from build123d import *

# Parameters (mm, degrees)
F0_R     = 3
F1_DEPTH = 1.5
F2_R     = 7.655
F2_W     = 13
F2_H     = 3
F3_DEPTH = 56.3
F4_R     = 2.93
F5_DEPTH = 26.25
F7_DEPTH = 18
F8_R     = 3
F9_DEPTH = 9.156


with BuildPart() as f1:
    # F0 (on Top) → F1 (new body, symmetric)
    with BuildSketch(Plane.XY):
        with BuildLine():
            Line((-2.85, -6.5), (9.35, -6.5))
            Line((9.35, -6.5), (9.35, 6.5))
            Line((9.35, 6.5), (-2.85, 6.5))
            ThreePointArc((-2.85, 6.5), (-9.35, 0), (-2.85, -6.5))
        make_face()
        with Locations((-2.85, 0)):
            Circle(F0_R, mode=Mode.SUBTRACT)
    extrude(amount=F1_DEPTH, both=True)

    # F2 (on face) → F3 (join)
    with BuildSketch(Plane.YZ.offset(9.35)):
        Circle(F2_R)
        Rectangle(F2_W, F2_H, mode=Mode.SUBTRACT)
        Rectangle(F2_W, F2_H)
    extrude(amount=F3_DEPTH)

    # F4 (on face) → F5 (join)
    with BuildSketch(Plane.YZ.offset(65.65)):
        Circle(F4_R)
    extrude(amount=F5_DEPTH)

    # F6 (on face) → F7 (join)
    with BuildSketch(Plane.YZ.offset(91.9)):
        with BuildLine():
            Line((2.516923, -1.5), (6.44, -1.5))
            Line((6.44, -1.5), (6.44, 1.5))
            Line((6.44, 1.5), (2.516923, 1.5))
            ThreePointArc((2.516923, 1.5), (2.824844, 0.777919), (2.93, 0))
            ThreePointArc((2.93, 0), (2.824844, -0.777919), (2.516923, -1.5))
        make_face()
        with BuildLine():
            Line((-2.516923, -1.5), (2.516923, -1.5))
            ThreePointArc((2.516923, -1.5), (2.824844, -0.777919), (2.93, 0))
            ThreePointArc((2.93, 0), (2.824844, 0.777919), (2.516923, 1.5))
            Line((2.516923, 1.5), (-2.516923, 1.5))
            ThreePointArc((-2.516923, 1.5), (-2.93, 0), (-2.516923, -1.5))
        make_face()
        with BuildLine():
            Line((-6.44, -1.5), (-2.516923, -1.5))
            ThreePointArc((-2.516923, -1.5), (-2.93, 0), (-2.516923, 1.5))
            Line((-2.516923, 1.5), (-6.44, 1.5))
            Line((-6.44, 1.5), (-6.44, -1.5))
        make_face()
    extrude(amount=F7_DEPTH)

    # F8 (on face) → F9 (cut, through all)
    with BuildSketch(Plane.XY.offset(1.5)):
        with Locations((103.46, 0)):
            Circle(F8_R)
        with BuildLine():
            ThreePointArc((103.46, 6.44), (108.013768, 4.553768), (109.9, 0))
            Line((109.9, 0), (109.9, 6.44))
            Line((109.9, 6.44), (103.46, 6.44))
        make_face()
        with BuildLine():
            ThreePointArc((109.9, 0), (108.013768, -4.553768), (103.46, -6.44))
            Line((103.46, -6.44), (109.9, -6.44))
            Line((109.9, -6.44), (109.9, 0))
        make_face()
    extrude(amount=-F9_DEPTH, mode=Mode.SUBTRACT)


solid = f1.part
Work out the finished part from the listing and answer in its coordinate system (mm). A direction names the side the tool comes from. Coordinates: 2 decimals unless noted, no trailing zeros. Order: outer loops, then holes, each group sorted by start corner. A loop starts at its lowest first (then second) coordinate and runs counter-clockwise, first axis right, second up. Notation, with made-up numbers: (-39, 24) - (-22, 24) arc R8 cw to (-22, 34) - close; hole circle Ø6 at (50.25, 63). An arc over 180 degrees is marked (long way). Put each result on its own line as item: value. Start each with the question number.
1) Find section A-A (y = 4). Give the vertices of the cut face in (x, z).
2) For faces 4 (the cylindrical face through (78.59, -0.64, -2.86)), 5 (the flat face through (3, 6.5, 0)), 6 (the flat face through (3, -6.5, 0)), 7 (the flat face through (98, -6.44, 0)), 8 (the flat face through (2, 0, 1.5)), determine the directions among +Z, -Z, +X, -X, +Y, -Y from which every point of the face is accessible in a straight line to the end or side of a thin tool.
3) Find section D-D (x = 62). Give the vertices of the cut face in (y, z) (3 decimals), plus the area to 3 significant figures.
4) Flat-ended cylindrical pins translate along their axes: pin 1 (3.5 mm diameter, centred on x = 0.5, z = 0, fed in from -Y); pin 2 (0.9 mm diameter, centred on x = 98.5, z = -0.5, fed in from +Y); pin 3 (6 mm diameter, centred on y = 5, z = 4, fed in from +X); pin 4 (3.5 mm diameter, centred on x = -2.85, y = 0, fed in from +Z). Find the tip coordinate at first contact, or state that the pin passes through.
5) Find the intervals of material crossed by line 1 (Y direction, x = -2.85, z = 0.65); line 2 (Y direction, x = 103.46, z = -0.35); line 3 (X direction, y = 2.5, z = -0.5), in increasing order. Write a range as from..to.
6) Find section C-C (x = 93). Give the vertices of the cut face in (y, z).
7) For a pull along Y with two mould halves and no side action, classify faces 1 (the cylindrical face through (37.106, -1.659, -7.473)), 2 (the cylindrical face through (0.01, 0.9, -0.02)), 3 (the flat face through (91.9, 4, 0)) as released by +Y, released by -Y, zero draft, split by the parting line, or undercut.
8) Find section B-B (z = 0). Give the vertices of the cut face in (x, y) (3 decimals).
Results list:
1. outline: (-7.97, -1.5) - (9.35, -1.5) - (9.35, -6.53) - (65.65, -6.53) - (65.65, 6.53) - (9.35, 6.53) - (9.35, 1.5) - (-7.97, 1.5) - close; (91.9, -1.5) - (108.51, -1.5) - (108.51, 1.5) - (91.9, 1.5) - close
2. face 4: none
2. face 5: +Z, -Z, -X, +Y
2. face 6: +Z, -Z, -X, -Y
2. face 7: +Z, -Z, +X, -Y
2. face 8: +Z, -X, +Y, -Y
3. outline: circle Ø15.31 at (0, 0)
3. area: 184 mm^2
4. pin 1: stops at y = -6.5
4. pin 2: stops at y = 6.44
4. pin 3: stops at x = 108.97
4. pin 4: passes through
5. line 1: y = -6.5..-3, 3..6.5
5. line 2: y = -6.44..-3, 3..6.44
5. line 3: x = -8.85..-4.51, -1.19..101.8, 105.12..109.39
6. outline: (-6.44, -1.5) - (6.44, -1.5) - (6.44, 1.5) - (-6.44, 1.5) - close
7. face 1: split by the parting line
7. face 2: undercut
7. face 3: zero draft
8. outline: (-2.85, -6.5) - (9.35, -6.5) - (9.35, -7.655) - (65.65, -7.655) - (65.65, -2.93) - (91.9, -2.93) - (91.9, -6.44) - (103.46, -6.44) arc R6.44 ccw to (109.9, 0) arc R6.44 ccw to (103.46, 6.44) - (91.9, 6.44) - (91.9, 2.93) - (65.65, 2.93) - (65.65, 7.655) - (9.35, 7.655) - (9.35, 6.5) - (-2.85, 6.5) arc R6.5 ccw to start; hole circle Ø6 at (-2.85, 0); hole circle Ø6 at (103.46, 0)
